from build123d import *

# Parameters (mm, degrees)
BOSS_EXTRUDE1_DEPTH = 20
SKETCH2_R           = 1.48
CUT_EXTRUDE1_DEPTH  = 3


with BuildPart() as part:
    # Sketch1 → Boss-Extrude1 (new body)
    with BuildSketch(Plane(origin=(0, 0, 0), x_dir=(1, 0, 0), z_dir=(0, 1, 0))):
        Polygon((-11, 0), (-11, 12), (11, 12), (11, -12), (-11, -12), align=None)
        with BuildLine():
            Line((-8, 6.532500515), (-8, -6.467499485))
            ThreePointArc((-8, -6.467499485), (0, -10.287300403), (8, -6.467499485))
            Line((8, -6.467499485), (8, 6.532500515))
            ThreePointArc((8, 6.532500515), (0, 10.328289451), (-8, 6.532500515))
        make_face(mode=Mode.SUBTRACT)
    extrude(amount=BOSS_EXTRUDE1_DEPTH)

    # Sketch2 → Cut-Extrude1 (cut)
    with BuildSketch(Plane(origin=(11, 0, 0), x_dir=(0, 0, -1), z_dir=(1, 0, 0))):
        with Locations((-9.6, 18)):
            Circle(SKETCH2_R)
        with Locations((9.6, 18)):
            Circle(SKETCH2_R)
        with Locations((9.6, 2)):
            Circle(SKETCH2_R)
        with Locations((-9.6, 2)):
            Circle(SKETCH2_R)
    extrude(amount=-CUT_EXTRUDE1_DEPTH, mode=Mode.SUBTRACT)


solid = part.part
For this review, take the finished solid that the model builds, in its own axes (mm). A direction names the side the tool comes from. Coordinates: 2 decimals unless noted, no trailing zeros. Order: outer loops, then holes, each group sorted by start corner. A loop starts at its lowest first (then second) coordinate and runs counter-clockwise, first axis right, second up. Notation, with made-up numbers: (22, 16) - (70, 16) arc R9 cw to (70, 28) - close; hole circle Ø8 at (-9.5, 75). An arc over 180 degrees is marked (long way). Use one line per item in the form item = value.
Q1. Consider section A-A (z = -0.5). Give the boundary of the cut face in (x, y).
Checked values:
outline = (-11, 0) - (-8, 0) - (-8, 20) - (-11, 20) - close; (8, 0) - (11, 0) - (11, 20) - (8, 20) - close
Q2. Consider section D-D (z = 9.6). Give the boundary of the cut face in (x, y), then the cut area to 3 significant figures.
Checked values:
outline = (-11, 0) - (-3.7, 0) - (-3.7, 20) - (-11, 20) - close; (3.7, 0) - (11, 0) - (11, 0.52) - (8, 0.52) - (8, 3.48) - (11, 3.48) - (11, 16.52) - (8, 16.52) - (8, 19.48) - (11, 19.48) - (11, 20) - (3.7, 20) - close
area = 274 mm2
Q3. Draft analysis for pull direction Z (two halves, no side actions). For faces 1 (the cylindrical face through (-0.128, 9.86, 10.287)), 2 (the cylindrical face through (9.521, 16.687, -10.283)), 3 (the flat face through (0, 10, 12)), 4 (the flat face through (10, 20, 0)), state which applies: +Z half, -Z half, draft (parallel to the pull), parting line (faces both ways), or undercut.
Checked values:
face_1 = undercut
face_2 = undercut
face_3 = +Z half
face_4 = draft
Q4. Consider section B-B (y = 2). Give the boundary of the cut face in (x, z), then the cut area to 3 significant figures.
Checked values:
outline = (-11, -12) - (11, -12) - (11, -11.08) - (8, -11.08) - (8, -8.12) - (11, -8.12) - (11, 8.12) - (8, 8.12) - (8, 11.08) - (11, 11.08) - (11, 12) - (-11, 12) - close; hole (-8, -6.53) arc R10.33 ccw to (8, -6.53) - (8, 6.47) arc R10.29 ccw to (-8, 6.47) - close
area = 217 mm2
Q5. For faces 5 (the flat face through (8, 2, -10)), 6 (the flat face through (8, 10, 0)), 7 (the flat face through (11, 10, 0)), list the 3-axis set-ups (+Z, -Z, +X, -X, +Y, -Y) from which the entire face can be reached by the end or side of a thin tool; tool diameter is ignored.
Checked values:
face_5 = +X
face_6 = +Y, -Y
face_7 = +Z, -Z, +X, +Y, -Y
Q6. For probe 1 along Y at (x, z) = (9.55, -9.6); probe 2 along X at (y, z) = (15.75, 2.5); probe 3 along Z at (x, y) = (3, 14.5), list the stretches that pass through material, from the lowest coordinate up. Write a range as from..to.
Checked values:
probe_1 = 0..0.52, 3.48..16.52, 19.48..20
probe_2 = -11..-8, 8..11
probe_3 = -12..-9.88, 9.84..12
Q7. Consider section C-C (x = 5). Give the boundary of the cut face in (y, z), then the cut area to 3 significant figures.
Checked values:
outline = (0, -12) - (20, -12) - (20, -9.04) - (0, -9.04) - close; (0, 8.99) - (20, 8.99) - (20, 12) - (0, 12) - close
area = 119 mm2
Q8. For P1, Ø6, axis at x = 7.5, z = -5.5, coming from the +Y side; P2, Ø2.5, axis at y = 18, z = 9.6, coming from the +X side, all flat-tipped, find the tip position at first contact; note any pin that passes through.
Checked values:
P1 = 20
P2 = 8
